Could you check a few things on this model? Use its own coordinates, in mm. A direction names the side the tool comes from. Give positions to 0.01 mm unless a question says otherwise; leave off trailing zeros. Write each loop counter-clockwise with the first axis right and the second up, starting at its lowest first coordinate (ties: lowest second). Pieces come first, ordered by that corner, then holes. Notation, with made-up numbers: M 54.25,51 L 102.25,51 A36 cw 102.25,89 Z; hole C -28.5,82.25 d1. An arc over 180 degrees is marked long. One line per item, written item: value.
```python
from build123d import *

# Parameters (mm, degrees)
SKETCH_1_R          = 17.5
SKETCH_2_R          = 25
SKETCH_3_R          = 6.5
CUT_EXTRUDE_1_DEPTH = 11
CUT_EXTRUDE_2_REACH = 17
SKETCH_4_R          = 4
FILLET_1_R          = 5


with BuildPart() as part:
    # 草图1 → 放样1 section 0
    with BuildSketch(Plane(origin=(0, 26, 0), x_dir=(-1, 0, 0), z_dir=(0, -1, 0))):
        Circle(SKETCH_1_R)
    # 草图2 → 放样1 section 1
    with BuildSketch(Plane(origin=(0, 0, 0), x_dir=(1, 0, 0), z_dir=(0, 1, 0))):
        Circle(SKETCH_2_R)
    loft()

    # 草图3 → 切除-拉伸1 (cut)
    with BuildSketch(Plane(origin=(0, 26, 0), x_dir=(1, 0, 0), z_dir=(0, 1, 0))):
        Circle(SKETCH_3_R)
    extrude(amount=-CUT_EXTRUDE_1_DEPTH, mode=Mode.SUBTRACT)

    # 草图4 → 切除-拉伸2 (cut, up to next)
    with BuildSketch(Plane(origin=(0, 15, 0), x_dir=(1, 0, 0), z_dir=(0, 1, 0)), mode=Mode.PRIVATE) as cut_extrude_2_sk1:
        Circle(SKETCH_4_R)
    cut_extrude_2_tool1 = extrude(cut_extrude_2_sk1.sketch, amount=-CUT_EXTRUDE_2_REACH, mode=Mode.PRIVATE) & part.part
    add(cut_extrude_2_tool1.solids().sort_by_distance((0, 15, 0))[0], mode=Mode.SUBTRACT)

    # 圆角1
    fillet_1_edges = [part.edges().sort_by_distance(p)[0] for p in [
        (17.5, 26, 0),
    ]]
    fillet(fillet_1_edges, radius=FILLET_1_R)


solid = part.part
```
1) We'd pull the mould along Z, two halves only. Please class faces 1 (the face through (0, 0, 5)), 2 (the face through (-5.158, 20.577, 3.955)), 3 (the face through (4.418, 16.011, 19.897)): pulls with the +Z half, pulls with the -Z half, needs draft (parallel to the pull), parting line crosses it, or undercut.
Outcome:
face 1: needs draft
face 2: undercut
face 3: parting line crosses it
2) I'm going to push flat-ended pins straight in: pin 1 (12 mm diameter, centred on x = -9, y = 8, fed in from +Z); pin 2 (6 mm diameter, centred on x = 14, z = -11.5, fed in from +Y); pin 3 (5 mm diameter, centred on x = 18, y = 16, fed in from +Z); pin 4 (6.5 mm diameter, centred on x = 0, z = 0, fed in from -Y). Where does each tip first touch, or does it pass through?
Outcome:
pin 1: stops at z = 23.46
pin 2: stops at y = 25.81
pin 3: stops at z = 13.44
pin 4: passes through
3) On a 3-axis mill with a long thin cutter (end or side, diameter ignored), from which of +Z, -Z, +X, -X, +Y, -Y can I reach the whole of each face in a straight line? I mean faces 4 (the face through (3, 15, -3)), 5 (the face through (-0.867, 7.605, 3.905)). Say none if no direction works.
Outcome:
face 4: +Y
face 5: +Y, -Y
4) If we section it at A-A, the plane x = 0: Write out the boundary of the cut face in (y, z).
Outcome:
outline: M 0,-25 L 22.39,-18.54 A5 ccw 26,-13.74 L 26,-6.5 L 15,-6.5 L 15,-4 L 0,-4 Z; M 0,4 L 15,4 L 15,6.5 L 26,6.5 L 26,13.74 A5 ccw 22.39,18.54 L 0,25 Z
5) If we section it at B-B, the plane y = 23.5: Write out the boundary of the cut face in (x, z).
Outcome:
outline: C 0,0 d36.14; hole C 0,0 d13
6) If we section it at C-C, the plane y = 4.5: Write out the boundary of the cut face in (x, z).
Outcome:
outline: C 0,0 d47.4; hole C 0,0 d8
7) Please list where these lines run through material, in increasing order: L1, parallel to X at y = 12, z = 0; L2, parallel to Z at x = 0, y = 6.25; L3, parallel to X at y = 20.5, z = 0. Write a range as from..to.
Outcome:
L1: x = -21.54..-4, 4..21.54
L2: z = -23.2..-4, 4..23.2
L3: x = -19.09..-6.5, 6.5..19.09
